Design review of the part built by this model. Coordinates are the model's own, in mm. A direction names the side the tool comes from. Coordinates: 2 decimals unless noted, no trailing zeros. Loops run counter-clockwise (first coordinate to the right, second up) from the corner with the lowest first, then second, coordinate; pieces in that order, holes last.
Q1. Add section C-C on x = 1. Give the number of separate pieces and of enclosed holes in the cut face, and give its area (3 significant figures).
Q2. Add section D-D on x = -3.25. Give the boundary of the cut face in (y, z) (1 decimal), and give its area (3 significant figures).
Q3. For P1, Ø4, axis at y = 22.225, z = 0, coming from the +X side; P2, Ø2, axis at x = 2.5, z = 15, coming from the +Y side; P3, Ø2, axis at x = 2.5, y = 6, coming from the +Z side; P4, Ø2, axis at x = -1.5, z = -11.5, coming from the -Y side, all flat-tipped, find the tip position at first contact; note any pin that passes through.
Q4. Draft analysis for pull direction Z (two halves, no side actions). For faces 1 (the face through (-4.762, -7, -13)), 2 (the face through (-3.153, 19.261, 21.005)), 3 (the face through (-0.067, -0.628, -14.274)), state which applies: released by +Z, released by -Z, zero draft, split by the parting line, or undercut.
Q5. Wall thickness on probe 1 along Y at (x, z) = (1, 0); probe 2 along Y at (x, z) = (-2.5, 0); probe 3 along X at (y, z) = (-14, 26.5): over which ranges is each line inside the solid? List them lowest first.
Q6. Machinability: for faces 4 (the face through (-1.588, 27, 11)), 5 (the face through (0.07, 0.75, 19.85)), which of the approach directions +Z, -Z, +X, -X, +Y, -Y give a long, thin tool a straight path to every point of the face, cutting with its end or side? Answer none if there is none.
Q7. Add section A-A on y = 0. Give the boundary of the cut face in (x, z).
```python
from build123d import *

# Parameters (mm, degrees)
SKETCH1_R           = 31.75
SKETCH1_R_2         = 14.2875
BOSS_EXTRUDE1_DEPTH = 4.7625
CUT_EXTRUDE1_START  = 3.175
SKETCH2_R           = 31.75
SKETCH2_R_2         = 28.4988
CUT_EXTRUDE1_DEPTH  = 3.175
SKETCH3_R           = 2.4892
CUT_EXTRUDE2_DEPTH  = 46.900442536
CHAMFER1_SIZE       = 1.5875


with BuildPart() as part:
    # Sketch1 → Boss-Extrude1 (new, symmetric)
    with BuildSketch(Plane(origin=(0, 0, 0), x_dir=(0, 0, -1), z_dir=(1, 0, 0))):
        with Locations(Location((0, 0, 0), (0, 0, 180))):
            Circle(SKETCH1_R)
        with Locations(Location((0, 0, 0), (0, 0, 180))):
            Circle(SKETCH1_R_2, mode=Mode.SUBTRACT)
    extrude(amount=BOSS_EXTRUDE1_DEPTH, both=True)

    # Sketch2 → Cut-Extrude1 (cut)
    with BuildSketch(Plane(origin=(-4.7625, 0, 0), x_dir=(0, 0, -1), z_dir=(1, 0, 0)).offset(CUT_EXTRUDE1_START)):
        with Locations(Location((0, 0, 0), (0, 0, 180))):
            Circle(SKETCH2_R)
        Circle(SKETCH2_R_2, mode=Mode.SUBTRACT)
    extrude(amount=-CUT_EXTRUDE1_DEPTH, mode=Mode.SUBTRACT)

    # Sketch3 → Cut-Extrude2 (cut, through all)
    with BuildSketch(Plane(origin=(4.7625, 0, 0), x_dir=(0, 0, -1), z_dir=(1, 0, 0))):
        with Locations((0, 22.225)):
            Circle(SKETCH3_R)
        with Locations((-22.225, 0)):
            Circle(SKETCH3_R)
        with Locations((0, -22.225)):
            Circle(SKETCH3_R)
        with Locations((22.225, 0)):
            Circle(SKETCH3_R)
    extrude(amount=-CUT_EXTRUDE2_DEPTH, mode=Mode.SUBTRACT)

    # Chamfer1
    chamfer1_edges = [part.edges().sort_by_distance(p)[0] for p in [
        (-1.5875, 0, -31.75),
    ]]
    chamfer(chamfer1_edges, length=CHAMFER1_SIZE)


solid = part.part
```
Entries:
1. separate pieces: 1
1. enclosed holes: 5
1. area: 2,450 mm2
2. outline: circle Ø57 at (0, 0); hole circle Ø5 at (-22.2, 0); hole circle Ø28.6 at (0, 0); hole circle Ø5 at (0, -22.2); hole circle Ø5 at (0, 22.2); hole circle Ø5 at (22.2, 0)
2. area: 1,830 mm2
3. P1: passes through
3. P2: stops at y = 28.5
3. P3: stops at z = 31.35
3. P4: stops at y = -29.13
4. face 1: zero draft
4. face 2: split by the parting line
4. face 3: undercut
5. probe 1: y = -31.75 to -24.71, -19.74 to -14.29, 14.29 to 19.74, 24.71 to 31.75
5. probe 2: y = -28.5 to -24.71, -19.74 to -14.29, 14.29 to 19.74, 24.71 to 28.5
5. probe 3: x = -1.59 to 4.76
6. face 4: -X
6. face 5: +X, -X
7. outline: (-4.76, -28.5) - (-1.59, -28.5) - (-1.59, -30.16) - (0, -31.75) - (4.76, -31.75) - (4.76, -24.71) - (-4.76, -24.71) - close; (-4.76, -19.74) - (4.76, -19.74) - (4.76, -14.29) - (-4.76, -14.29) - close; (-4.76, 14.29) - (4.76, 14.29) - (4.76, 19.74) - (-4.76, 19.74) - close; (-4.76, 24.71) - (4.76, 24.71) - (4.76, 31.75) - (0, 31.75) - (-1.59, 30.16) - (-1.59, 28.5) - (-4.76, 28.5) - close
